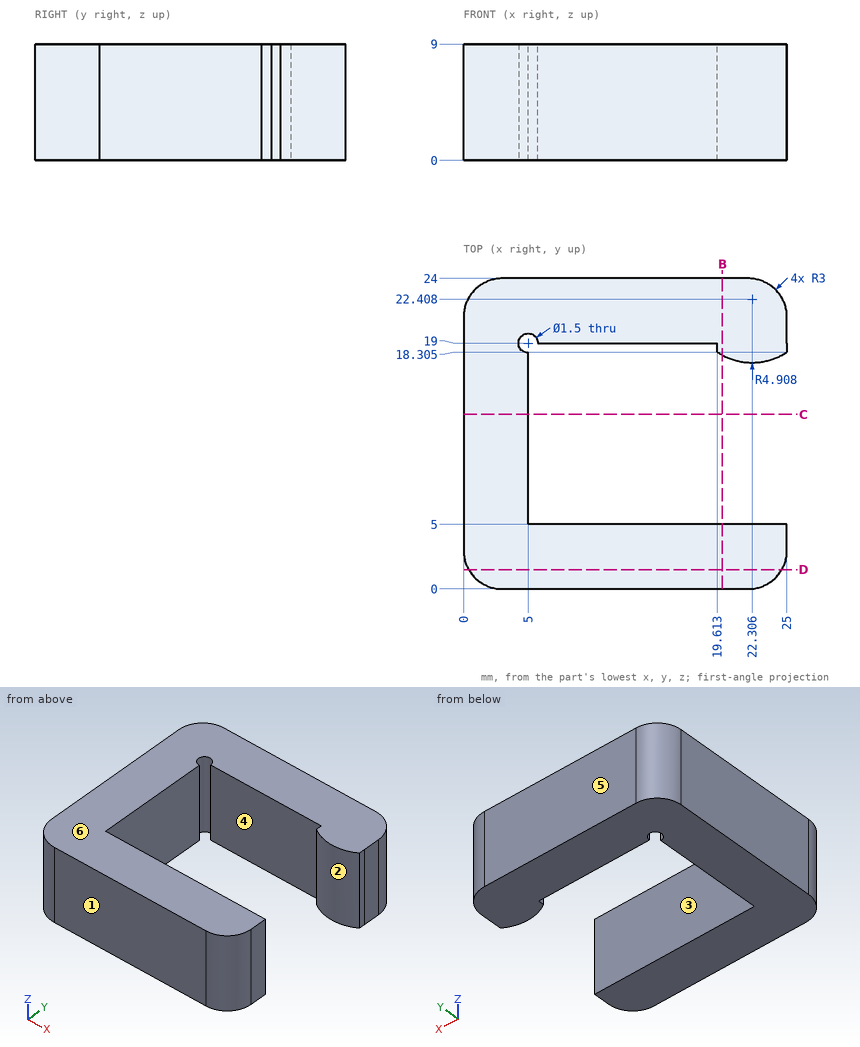
Verification items for this drawing (mm, ordinates from the low corner). A direction names the side the tool comes from. Coordinates: 2 decimals unless noted, no trailing zeros. Loops run counter-clockwise (first coordinate to the right, second up) from the corner with the lowest first, then second, coordinate; pieces in that order, holes last. Notation, with made-up numbers: (-23.75, 47) -> (-19.75, 47) arc R19 cw to (-19.75, 78) -> close; hole circle Ø5 at (-4, -0.5). An arc over 180 degrees is marked (long way). Answer in a Markdown table with one row per item. Add a question column.
1. Access from +Z, -Z, +X, -X, +Y, -Y to the whole of each face (thin tool, end or side, straight path). Record for the marked faces 1, 2 and 3.
2. Section check D-D, the plane y = 1.5. Enter the section's corners in (x, z).
3. Draft check along Y on the marked faces 4, 5 and 6. Enter one of: +Y half, -Y half, draft (parallel to the pull), parting line (faces both ways), or undercut.
4. Section check C-C, the plane y = 13.5. Enter the section's corners in (x, z), then the cut area to 3 significant figures.
5. Material ranges on probe 1 along Y at (x, z) = (13, 8); probe 2 along Y at (x, z) = (21, 3.75); probe 3 along X at (y, z) = (12, 6.25), recorded low to high. Write a range as [from, to].
6. Depth check by flat-ended pin: P1, Ø1.9, axis at x = 5, y = 19, coming from the -Z side. Enter the tip coordinate at first touch or a pass-through.
7. Section check B-B, the plane x = 20. Enter the section's corners in (y, z) (1 decimal).
Derived:
| question | item | result |
|---|---|---|
| 1 | face 1 | +Z, -Z, +X, -X, -Y |
| 1 | face 2 | +Z, -Z |
| 1 | face 3 | +Z, -Z, +X |
| 2 | outline | (0.4, 0) -> (24.6, 0) -> (24.6, 9) -> (0.4, 9) -> close |
| 3 | face 4 | undercut |
| 3 | face 5 | +Y half |
| 3 | face 6 | draft |
| 4 | outline | (0, 0) -> (5, 0) -> (5, 9) -> (0, 9) -> close |
| 4 | area | 45.0 mm² |
| 5 | probe 1 | y = [0, 5], [19, 24] |
| 5 | probe 2 | y = [0, 5], [17.68, 24] |
| 5 | probe 3 | x = [0, 5] |
| 6 | P1 | stops at z = 0 |
| 7 | outline | (0, 0) -> (5, 0) -> (5, 9) -> (0, 9) -> close; (18.1, 0) -> (24, 0) -> (24, 9) -> (18.1, 9) -> close |
